Geometry check sheet. Reference: drawing and pictorial views, mm from the part's lowest x, y, z. A direction names the side the tool comes from. Give positions to 0.01 mm unless a question says otherwise; leave off trailing zeros. Write each loop counter-clockwise with the first axis right and the second up, starting at its lowest first coordinate (ties: lowest second). Pieces come first, ordered by that corner, then holes. Notation, with made-up numbers: (-38.5, 32) - (-29.5, 32) arc R7 ccw to (-29.5, 44) - close; hole circle Ø11 at (-24.75, 32.25). An arc over 180 degrees is marked (long way). Write item = value, one per line. Start each with the question number.
(1) Depth check by flat-ended pin: pin 1 Ø10 at (y, z) = (17.5, 32.5) entering from +X; pin 2 Ø1.5 at (x, z) = (34.5, 44) entering from -Y; pin 3 Ø1.5 at (y, z) = (26, 10) entering from -X. Enter the tip coordinate at first touch or a pass-through.
(2) Section check A-A, the plane z = 14. Enter the section's corners in (x, y) (1 decimal).
(3) Section check B-B, the plane x = 41. Enter the section's corners in (y, z) (1 decimal).
(4) Section check C-C, the plane y = 33. Enter the section's corners in (x, z).
(5) Access from +Z, -Z, +X, -X, +Y, -Y to the whole of each face (thin tool, end or side, straight path). Record for the marked faces 1, 2 and 3.
(6) Thickness scan on L1, parallel to Y at x = 44, z = 3 (1 decimal); L2, parallel to Z at x = 52, y = 12; L3, parallel to X at y = 11.5, z = 14. Record the ranges inside material, lowest first.
(7) Section check D-D, the plane x = 5. Enter the section's corners in (y, z) (1 decimal).
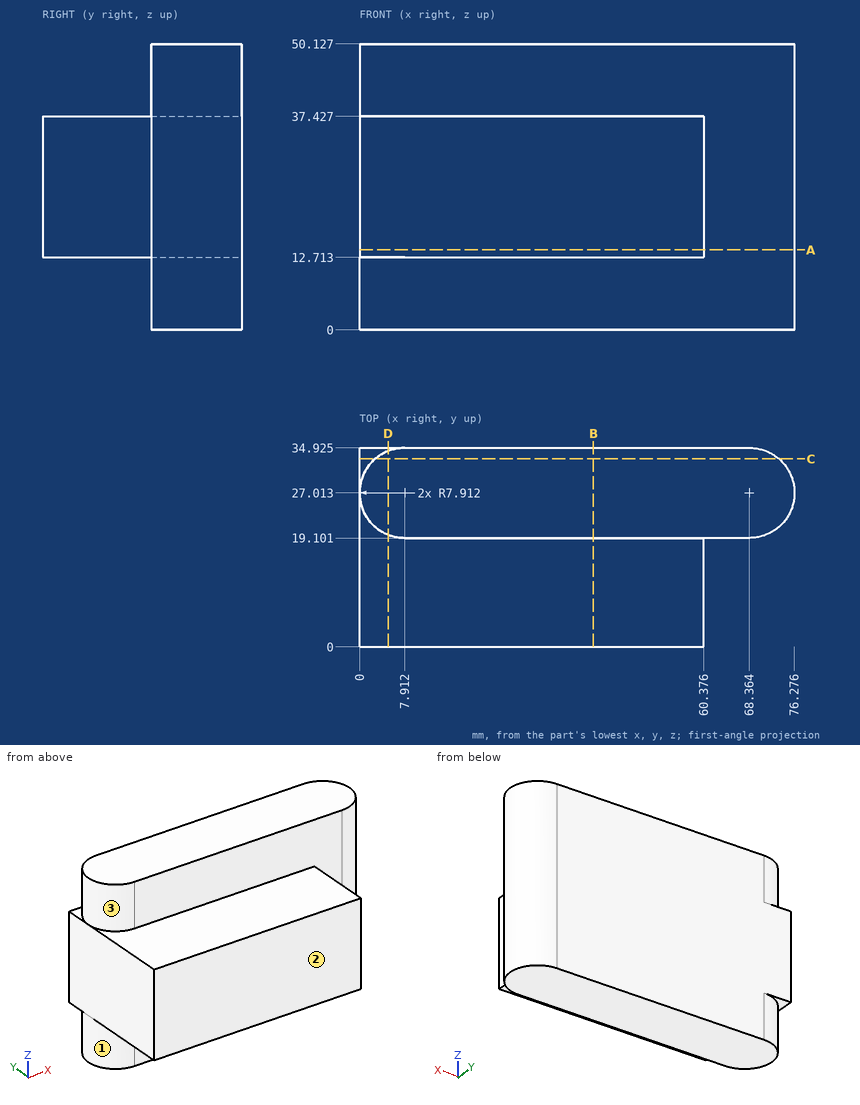
Model answer:
q1.pin_1 = 74.86
q1.pin_2 = 19.1
q1.pin_3 = 0
q2.outline = (0, 0) - (60.4, 0) - (60.4, 19.1) - (68.4, 19.1) arc R7.9 ccw to (68.4, 34.9) - (0, 34.9) - close
q3.outline = (0, 12.7) - (19.1, 12.7) - (19.1, 0) - (34.9, 0) - (34.9, 50.1) - (19.1, 50.1) - (19.1, 37.4) - (0, 37.4) - close
q4.outline = (0, 12.71) - (2.74, 12.71) - (2.74, 0) - (73.54, 0) - (73.54, 50.13) - (2.74, 50.13) - (2.74, 37.43) - (0, 37.43) - close
q5.face_1 = -Z, -X
q5.face_2 = +Z, -Z, +X, -X, -Y
q5.face_3 = +Z, -X
q6.L1 = 19.1 to 34.9
q6.L2 = 12.71 to 37.43
q6.L3 = 0 to 60.38
q7.outline = (0, 12.7) - (19.7, 12.7) - (19.7, 0) - (34.4, 0) - (34.4, 12.7) - (34.9, 12.7) - (34.9, 37.4) - (34.4, 37.4) - (34.4, 50.1) - (19.7, 50.1) - (19.7, 37.4) - (0, 37.4) - close
